Build history of the part. All positions in model axes, mm. A direction names the side the tool comes from. Give positions to 0.01 mm unless a question says otherwise; leave off trailing zeros. Order: outer loops, then holes, each group sorted by start corner. A loop starts at its lowest first (then second) coordinate and runs counter-clockwise, first axis right, second up. Notation, with made-up numbers: (17.5, 79.25) - (38.5, 79.25) arc R28 ccw to (38.5, 112.25) - close; hole circle Ø4 at (-30, 88). An arc over 180 degrees is marked (long way). Write each question's results on one line, items separated by ' | '. Start each with the question number.
from build123d import *

# Parameters (mm, degrees)
SKETCH1_W                      = 86.55
SKETCH1_H                      = 17.1
BOSS_EXTRUDE1_DEPTH            = 14
SKETCH2_W                      = 88.55
SKETCH2_H                      = 17.1
BOSS_EXTRUDE2_DEPTH            = 23.55
SKETCH3_W                      = 37.55
SKETCH3_H                      = 17.1
BOSS_EXTRUDE3_DEPTH            = 2
SKETCH4_W                      = 90.55
SKETCH4_H                      = 17.1
BOSS_EXTRUDE4_DEPTH            = 23.55
SKETCH5_W                      = 2
SKETCH5_H                      = 14
CUT_EXTRUDE1_DEPTH             = 3
CUT_EXTRUDE2_DEPTH             = 14.1
SKETCH7_W                      = 2
SKETCH7_H                      = 14
CUT_EXTRUDE3_DEPTH             = 2
BOSS_EXTRUDE5_DEPTH            = 5
SKETCH9_W                      = 87.55
SKETCH9_H                      = 19.1
CUT_EXTRUDE4_DEPTH             = 1.55
SKETCH10_W                     = 61.1
SKETCH10_H                     = 17.1
BOSS_EXTRUDE6_DEPTH            = 1
CUT_EXTRUDE5_REACH             = 79.588
SKETCH11_W                     = 87.55
SKETCH11_H                     = 19.1
SKETCH12_W                     = 13.7
SKETCH12_H                     = 9.8
CUT_EXTRUDE6_DEPTH             = 127.470668932
SKETCH13_W                     = 13.7
SKETCH13_H                     = 9.8
CUT_EXTRUDE7_DEPTH             = 127.470668932
SKETCH14_W                     = 14.3
SKETCH14_H                     = 10.2
CUT_EXTRUDE8_DEPTH             = 127.470668932
CUT_EXTRUDE10_DEPTH            = 78.587821209
CUT_EXTRUDE11_REACH            = 81.122
F_2_8_2_8_DIAMETER_HOLE1_D     = 2.8
F_6_2_6_2_DIAMETER_HOLE1_D     = 6.2
F_6_2_6_2_DIAMETER_HOLE1_DEPTH = 2
FILLET1_R                      = 1
FILLET2_R                      = 2
FILLET3_R                      = 2.55
FILLET4_R                      = 3.55


with BuildPart() as part:
    # Sketch1 → Boss-Extrude1 (new body)
    with BuildSketch(Plane.XY.offset(63.69)):
        with Locations((-0.775, 5.55)):
            Rectangle(SKETCH1_W, SKETCH1_H)
    extrude(amount=-BOSS_EXTRUDE1_DEPTH)

    # Sketch2 → Boss-Extrude2 (add)
    with BuildSketch(Plane(origin=(0, 0, 49.69), x_dir=(-1, 0, 0), z_dir=(0, 0, -1))):
        with Locations((-0.225, 5.55)):
            Rectangle(SKETCH2_W, SKETCH2_H)
    extrude(amount=BOSS_EXTRUDE2_DEPTH)

    # Sketch3 → Boss-Extrude3 (add)
    with BuildSketch(Plane(origin=(44.5, 0, 0), x_dir=(0, 0, -1), z_dir=(1, 0, 0))):
        with Locations((-44.915, 5.55)):
            Rectangle(SKETCH3_W, SKETCH3_H)
    extrude(amount=BOSS_EXTRUDE3_DEPTH)

    # Sketch4 → Boss-Extrude4 (add)
    with BuildSketch(Plane.XY.offset(63.69)):
        with Locations((1.225, 5.55)):
            Rectangle(SKETCH4_W, SKETCH4_H)
    extrude(amount=BOSS_EXTRUDE4_DEPTH)

    # Sketch5 → Cut-Extrude1 (cut)
    with BuildSketch(Plane.XZ.offset(3)):
        with Locations((45.5, 56.69)):
            Rectangle(SKETCH5_W, SKETCH5_H)
    extrude(amount=-CUT_EXTRUDE1_DEPTH, mode=Mode.SUBTRACT)

    # Sketch6 → Cut-Extrude2 (cut)
    with BuildSketch(Plane(origin=(0, 14.1, 0), x_dir=(-1, 0, 0), z_dir=(0, 1, 0))):
        Polygon((43.05, 29.69), (43.05, 83.69), (-44.5, 83.69), (-44.5, 63.69), (-42.5, 63.69), (-42.5, 49.69), (-44.5, 49.69), (-44.5, 29.69), align=None)
    extrude(amount=-CUT_EXTRUDE2_DEPTH, mode=Mode.SUBTRACT)

    # Sketch7 → Cut-Extrude3 (cut)
    with BuildSketch(Plane.XZ):
        with Locations((45.5, 56.69)):
            Rectangle(SKETCH7_W, SKETCH7_H)
    extrude(amount=-CUT_EXTRUDE3_DEPTH, mode=Mode.SUBTRACT)

    # Sketch8 → Boss-Extrude5 (add)
    with BuildSketch(Plane(origin=(0, 14.1, 0), x_dir=(-1, 0, 0), z_dir=(0, 1, 0))):
        with BuildLine():
            Line((-44.5, 83.69), (-44.5, 29.69))
            Line((-44.5, 29.69), (44.05, 29.69))
            ThreePointArc((44.05, 29.69), (43.303122292, 27.886877708), (41.5, 27.14))
            Line((41.5, 27.14), (-45.5, 27.14))
            Line((-45.5, 27.14), (-45.5, 86.24))
            Line((-45.5, 86.24), (41.5, 86.24))
            ThreePointArc((41.5, 86.24), (43.303122292, 85.493122292), (44.05, 83.69))
            Line((44.05, 83.69), (-44.5, 83.69))
        make_face()
    extrude(amount=BOSS_EXTRUDE5_DEPTH)

    # Sketch9 → Cut-Extrude4 (cut)
    with BuildSketch(Plane(origin=(0, 0, 83.69), x_dir=(-1, 0, 0), z_dir=(0, 0, -1))):
        with Locations((-0.725, 9.55)):
            Rectangle(SKETCH9_W, SKETCH9_H)
    extrude(amount=-CUT_EXTRUDE4_DEPTH, mode=Mode.SUBTRACT)

    # Sketch10 → Boss-Extrude6 (add)
    with BuildSketch(Plane.ZY.offset(44.05)):
        with Locations((56.69, 5.55)):
            Rectangle(SKETCH10_W, SKETCH10_H)
    extrude(amount=BOSS_EXTRUDE6_DEPTH)

    # Sketch11 → Cut-Extrude5 (cut, up to next)
    with BuildSketch(Plane(origin=(0, 0, 28.14), x_dir=(-1, 0, 0), z_dir=(0, 0, -1)), mode=Mode.PRIVATE) as cut_extrude5_sk1:
        with Locations((-0.725, 9.55)):
            Rectangle(SKETCH11_W, SKETCH11_H)
    cut_extrude5_tool1 = extrude(cut_extrude5_sk1.sketch, amount=-CUT_EXTRUDE5_REACH, mode=Mode.PRIVATE) & part.part
    add(cut_extrude5_tool1.solids().sort_by_distance((0.725, 9.55, 28.14))[0], mode=Mode.SUBTRACT)

    # Sketch12 → Cut-Extrude6 (cut, through all)
    with BuildSketch(Plane(origin=(-43.05, 0, 0), x_dir=(0, 0, -1), z_dir=(1, 0, 0))):
        with Locations((-75.705690784, 9.2)):
            Rectangle(SKETCH12_W, SKETCH12_H)
    extrude(amount=-CUT_EXTRUDE6_DEPTH, mode=Mode.SUBTRACT)

    # Sketch13 → Cut-Extrude7 (cut, through all)
    with BuildSketch(Plane(origin=(-43.05, 0, 0), x_dir=(0, 0, -1), z_dir=(1, 0, 0))):
        with Locations((-57.305690784, 9.2)):
            Rectangle(SKETCH13_W, SKETCH13_H)
    extrude(amount=-CUT_EXTRUDE7_DEPTH, mode=Mode.SUBTRACT)

    # Sketch14 → Cut-Extrude8 (cut, through all)
    with BuildSketch(Plane(origin=(-43.05, 0, 0), x_dir=(0, 0, -1), z_dir=(1, 0, 0))):
        with Locations((-38.80469145, 9)):
            Rectangle(SKETCH14_W, SKETCH14_H)
    extrude(amount=-CUT_EXTRUDE8_DEPTH, mode=Mode.SUBTRACT)

    # Sketch16 → Cut-Extrude10 (cut, through all)
    with BuildSketch(Plane.XY.offset(28.14)):
        Polygon((20.057791158, 10.08), (4.557791136, 10.08), (4.557791136, 6.52999997), (7.057791136, 4.02999997), (17.557791158, 4.02999997), (20.057791158, 6.52999997), align=None)
    extrude(amount=-CUT_EXTRUDE10_DEPTH, mode=Mode.SUBTRACT)

    # Sketch17 → Cut-Extrude11 (cut, up to next)
    with BuildSketch(Plane(origin=(0, 0, 26.14), x_dir=(-1, 0, 0), z_dir=(0, 0, -1)), mode=Mode.PRIVATE) as cut_extrude11_sk1:
        with BuildLine():
            Line((-36.3834392, 6.568002867), (-30.8834392, 6.568002867))
            ThreePointArc((-30.8834392, 6.568002867), (-29.3834392, 5.068002867), (-30.8834392, 3.568002867))
            Line((-30.8834392, 3.568002867), (-36.3834392, 3.568002867))
            ThreePointArc((-36.3834392, 3.568002867), (-37.8834392, 5.068002867), (-36.3834392, 6.568002867))
        make_face()
    cut_extrude11_tool1 = extrude(cut_extrude11_sk1.sketch, amount=-CUT_EXTRUDE11_REACH, mode=Mode.PRIVATE) & part.part
    add(cut_extrude11_tool1.solids().sort_by_distance((33.633439, 5.068003, 26.14))[0], mode=Mode.SUBTRACT)

    # Ø2.8 (2.8) Diameter Hole1 (through all)
    with Locations(Plane(origin=(0, 0, 0), x_dir=(1, 0, 0), z_dir=(0, 1, 0))):
        with Locations((40.75, -81.19), (40.75, -32.19), (-17.25, -32.19), (-17.25, -81.19)):
            Hole(F_2_8_2_8_DIAMETER_HOLE1_D / 2)

    # Ø6.2 (6.2) Diameter Hole1
    with Locations(Plane(origin=(0, 0, 26.14), x_dir=(-1, 0, 0), z_dir=(0, 0, -1))):
        with Locations((9.353475334, 6.6)):
            Hole(F_6_2_6_2_DIAMETER_HOLE1_D / 2, depth=F_6_2_6_2_DIAMETER_HOLE1_DEPTH)

    # Fillet1
    fillet1_edges = [part.edges().sort_by_distance(p)[0] for p in [
        (20.057791158, 10.08, 27.14),
        (20.057791158, 6.52999997, 27.14),
        (17.557791158, 4.02999997, 27.14),
        (7.057791136, 4.02999997, 27.14),
        (4.557791136, 6.52999997, 27.14),
        (4.557791136, 10.08, 27.14),
    ]]
    fillet(fillet1_edges, radius=FILLET1_R)

    # Fillet2
    fillet2_edges = [part.edges().sort_by_distance(p)[0] for p in [
        (42.5, -1.5, 49.69),
        (42.5, -1.5, 63.69),
        (-44.05, 4.3, 82.555690784),
        (45.5, 2, 63.69),
        (-44.05, 4.3, 64.155690784),
        (-43.05, 9.55, 85.24),
        (44.5, 9.55, 85.24),
        (-44.05, 4.3, 50.455690784),
        (45.5, 2, 49.69),
        (-44.05, 3.9, 45.95469145),
        (-44.05, 4.3, 68.855690784),
        (-44.05, 3.9, 31.65469145),
        (44.5, 9.55, 28.14),
        (-43.05, 9.55, 28.14),
    ]]
    fillet(fillet2_edges, radius=FILLET2_R)

    # Fillet3
    fillet3_edges = [part.edges().sort_by_distance(p)[0] for p in [
        (45.5, 16.6, 86.24),
        (45.5, 16.6, 27.14),
    ]]
    fillet(fillet3_edges, radius=FILLET3_R)

    # Fillet4
    fillet4_edges = [part.edges().sort_by_distance(p)[0] for p in [
        (-45.05, 5.55, 26.14),
        (-45.05, 5.55, 87.24),
        (46.5, 5.55, 26.14),
        (46.5, 5.55, 87.24),
    ]]
    fillet(fillet4_edges, radius=FILLET4_R)


solid = part.part
Item 1: Two-plate mould, pull along Z, no slides. Class faces 1 (the cylindrical face through (-44.06, 4.9, 69.43)), 2 (the flat face through (12, 4.03, 27)), 3 (the flat face through (1, 5, 26.14)), 4 (the cylindrical face through (-42.45, 9.68, 28.71)): +Z half, -Z half, draft (parallel to the pull), parting line (faces both ways), or undercut.
Item 2: Flat gauge pins, fed straight in: pin 1 Ø1 at (x, z) = (-44, 49) entering from +Y; pin 2 Ø2 at (x, y) = (-43.5, 10.5) entering from +Z; pin 3 Ø0.6 at (x, y) = (46, -2) entering from -Z (3 decimals); pin 4 Ø2 at (x, z) = (-17.25, 81.19) entering from -Y. Where does each tip first touch, or does it go through?
Item 3: Probe line 1 along X through (y, z) = (-0.25, 81); line 2 along Z through (x, y) = (-17.25, -2.1); line 3 along Z through (x, y) = (18, 2). List the from-to ranges inside material, lowest first. Write a range as from..to.
Item 4: Cut at D-D, the plane x = -34.5. List the corners of the cut face in (y, z), then the cut area to 3 significant figures.
Item 5: Cut at A-A, the plane x = 40.75. List the corners of the cut face in (y, z).
Item 6: Cut at C-C, the plane z = 75.5. List the corners of the cut face in (x, y).
Item 7: Cut at B-B, the plane y = 11.25. List the corners of the cut face in (x, z), then the cut area to 3 significant figures.
Item 8: Which spindle directions (+Z, -Z, +X, -X, +Y, -Y) get a long thin tool onto all of the face, cutting with end or side? Do faces 5 (the cylindrical face through (-44.064, 4.47, 45.353)), 6 (the cylindrical face through (-42, 10, 85)), 7 (the flat face through (12, 10.08, 27)), 8 (the cylindrical face through (40.9, -1.5, 30.8)). Say none if no direction does.
Values found:
1) face 1: undercut | face 2: draft | face 3: -Z half | face 4: undercut
2) pin 1: stops at y = 14.1 | pin 2: stops at z = 87.1 | pin 3: stops at z = 27.445 | pin 4: passes through
3) line 1: x = -45.05..-18.64, -15.86..39.36, 42.14..46.5 | line 2: z = 26.14..30.79, 33.59..79.79, 82.59..87.24 | line 3: z = 26.14..28.14, 85.24..87.24
4) outline: (-3, 26.14) - (14.1, 26.14) - (14.1, 27.14) - (19.1, 27.14) - (19.1, 28.14) - (0, 28.14) - (0, 85.24) - (19.1, 85.24) - (19.1, 86.24) - (14.1, 86.24) - (14.1, 87.24) - (-3, 87.24) - close | area: 250 mm2
5) outline: (-3, 26.14) - (14.1, 26.14) - (14.1, 27.14) - (19.1, 27.14) - (19.1, 28.14) - (0, 28.14) - (0, 30.79) - (-3, 30.79) - close; (-3, 33.59) - (0, 33.59) - (0, 79.79) - (-3, 79.79) - close; (-3, 82.59) - (0, 82.59) - (0, 85.24) - (19.1, 85.24) - (19.1, 86.24) - (14.1, 86.24) - (14.1, 87.24) - (-3, 87.24) - close
6) outline: (-45.05, -3) - (46.5, -3) - (46.5, 14.1) - (45.5, 14.1) - (45.5, 19.1) - (44.5, 19.1) - (44.5, 0) - (-43.05, 0) - (-43.05, 4.3) - (-45.05, 4.3) - close
7) outline: (-45.05, 29.69) arc R3.55 ccw to (-41.5, 26.14) - (42.95, 26.14) arc R3.55 ccw to (46.5, 29.69) - (46.5, 83.69) arc R3.55 ccw to (42.95, 87.24) - (-41.5, 87.24) arc R3.55 ccw to (-45.05, 83.69) - (-45.05, 82.56) - (-43.05, 82.56) - (-43.05, 83.24) arc R2 cw to (-41.05, 85.24) - (42.5, 85.24) arc R2 cw to (44.5, 83.24) - (44.5, 30.14) arc R2 cw to (42.5, 28.14) - (-41.05, 28.14) arc R2 cw to (-43.05, 30.14) - (-43.05, 31.65) - (-45.05, 31.65) - close; (-45.05, 45.95) - (-43.05, 45.95) - (-43.05, 50.46) - (-45.05, 50.46) - close; (-45.05, 64.16) - (-43.05, 64.16) - (-43.05, 68.86) - (-45.05, 68.86) - close | area: 504 mm2
8) face 5: -X, +Y | face 6: +Y | face 7: -Z | face 8: +Y, -Y
